```python
from build123d import *

# Parameters (mm, degrees)
F0_R     = 2.5
F1_DEPTH = 3


# Not quite as in the source:
# - a feature names something its author has since deleted; it is built from what else it names


with BuildPart() as f1:
    # F0 (on Top) → F1 (new body)
    with BuildSketch(Plane.XY):
        with BuildLine():
            Line((-14.8844467476, 9.0084131807), (-14.8591619832, 9.0084131807))
            Line((-14.8591619832, 9.0084131807), (5.1155532524, 9.0084131807))
            Line((5.1155532524, 9.0084131807), (6.5302648152, 10.8946952644))
            ThreePointArc((6.5302648152, 10.8946952644), (-4.8844467476, 10.0579512552), (-16.2991583104, 10.8946952644))
            Line((-16.2991583104, 10.8946952644), (-14.8844467476, 9.0084131807))
        make_face()
        Polygon((5.1155532524, 9.0084131807), (-14.8591619832, 9.0084131807), (-14.8591619832, -0.9915868193), (5.1408380168, -0.9915868193), (5.1408380168, 9.0084131807), align=None)
        with Locations((-4.8591619832, 3.7784131807)):
            Circle(F0_R, mode=Mode.SUBTRACT)
    extrude(amount=F1_DEPTH)


solid = f1.part
```
For this review, take the finished solid that the model builds, in its own axes (mm). A direction names the side the tool comes from. Round coordinates to 2 decimals unless told otherwise and drop trailing zeros. Write each loop counter-clockwise with the first axis right and the second up, starting at its lowest first coordinate (ties: lowest second). Pieces come first, ordered by that corner, then holes. Notation, with made-up numbers: (31, 56) -> (77, 56) arc R31 ccw to (77, 87) -> close; hole circle Ø6 at (-38, 2.25). An arc over 180 degrees is marked (long way). One line per question, with ' | ' between items. Start each with the question number.
(1) Insertion check: P1, Ø1, axis at y = 8.5, z = 1, coming from the +X side; P2, Ø1.5, axis at y = 5.5, z = 1.5, coming from the -X side. Each pin has a flat end and moves straight along its axis. Give the tip position at first contact, or say it passes through.
(2) Add section A-A, the plane y = 1.5. Write out the cut boundary in (x, z).
(3) Add section B-B, the plane x = -6. Write out the cut boundary in (y, z), plus the area to 3 significant figures.
(4) For line 1 along Y through (x, z) = (-4.75, 0.75); line 2 along X through (y, z) = (6.75, 1.25); line 3 along X through (y, z) = (2.5, 0.6), list the stretches that pass through material, from the lowest coordinate up. Write a range as from..to.
(5) Mouldability with a two-part tool opening along Y and no side actions: class faces 1 (the face through (-4.72, 10.06, 1.48)), 2 (the face through (-3.52, 5.89, 1.48)), 3 (the face through (5.141, 4, 1)) as released by +Y, released by -Y, zero draft, split by the parting line, or undercut.
(6) Add section D-D, the plane y = 0.25. Write out the cut boundary in (x, z).
(7) Tool access review of faces 4 (the face through (-14.859, 4, 1)), 5 (the face through (-5, -0.992, 1)): name each direction out of +Z, -Z, +X, -X, +Y, -Y from which nothing blocks a thin tool from reaching the whole face with its end or side.
Answer list:
1) P1: x = 5.14 | P2: x = -14.86
2) outline: (-14.86, 0) -> (-5.89, 0) -> (-5.89, 3) -> (-14.86, 3) -> close; (-3.83, 0) -> (5.14, 0) -> (5.14, 3) -> (-3.83, 3) -> close
3) outline: (-0.99, 0) -> (1.55, 0) -> (1.55, 3) -> (-0.99, 3) -> close; (6, 0) -> (10.07, 0) -> (10.07, 3) -> (6, 3) -> close | area: 19.8 mm²
4) line 1: -0.99..1.28, 6.28..10.06 | line 2: -14.86..5.14 | line 3: -14.86..-7.01, -2.71..5.14
5) face 1: released by +Y | face 2: undercut | face 3: zero draft
6) outline: (-14.86, 0) -> (5.14, 0) -> (5.14, 3) -> (-14.86, 3) -> close
7) face 4: +Z, -Z, -X, -Y | face 5: +Z, -Z, +X, -X, -Y
